Design review of the part built by this model. Coordinates are the model's own, in mm. A direction names the side the tool comes from. Give positions to 0.01 mm unless a question says otherwise; leave off trailing zeros. Order: outer loops, then holes, each group sorted by start corner. A loop starts at its lowest first (then second) coordinate and runs counter-clockwise, first axis right, second up. Notation, with made-up numbers: (42, -40) -> (50, -40) arc R17 ccw to (50, -33) -> close; hole circle Ø5 at (66.5, 56.5). An arc over 180 degrees is marked (long way). Return JSON: item names as keys, results as strings.
```python
from build123d import *

# Parameters (mm, degrees)
BOSS_EXTRUDE1_DEPTH = 176.53
BOSS_EXTRUDE2_DEPTH = 1.905


with BuildPart() as part:
    # Sketch2 → Boss-Extrude1 (new body)
    with BuildSketch(Plane.XY):
        with BuildLine():
            Line((-8.5725, 0), (8.5725, 0))
            ThreePointArc((8.5725, 0), (8.931710245, 0.148789755), (9.0805, 0.508))
            Line((9.0805, 0.508), (9.0805, 2.794))
            ThreePointArc((9.0805, 2.794), (8.931710245, 3.153210245), (8.5725, 3.302))
            Line((8.5725, 3.302), (5.9055, 3.302))
            Line((5.9055, 3.302), (5.9055, 2.5654))
            Line((5.9055, 2.5654), (7.8105, 2.5654))
            Line((7.8105, 2.5654), (7.8105, 1.2954))
            Line((7.8105, 1.2954), (-7.8105, 1.2954))
            Line((-7.8105, 1.2954), (-7.8105, 2.5654))
            Line((-7.8105, 2.5654), (-5.3975, 2.5654))
            Line((-5.3975, 2.5654), (-5.3975, 3.302))
            Line((-5.3975, 3.302), (-8.5725, 3.302))
            ThreePointArc((-8.5725, 3.302), (-8.931710245, 3.153210245), (-9.0805, 2.794))
            Line((-9.0805, 2.794), (-9.0805, 0.508))
            ThreePointArc((-9.0805, 0.508), (-8.931710245, 0.148789755), (-8.5725, 0))
        make_face()
    extrude(amount=-BOSS_EXTRUDE1_DEPTH)

    # Sketch3 → Boss-Extrude2 (add)
    with BuildSketch(Plane(origin=(0, 0, 0), x_dir=(1, 0, 0), z_dir=(0, 1, 0))):
        with BuildLine():
            Line((8.5725, 84.455), (8.5725, 92.075))
            ThreePointArc((8.5725, 92.075), (13.193617406, 88.265), (8.5725, 84.455))
        make_face()
    boss_extrude2 = extrude(amount=BOSS_EXTRUDE2_DEPTH)

    # Mirror1: Boss-Extrude2 across plane
    add(boss_extrude2.mirror(Plane(origin=(0, 0, 0), x_dir=(0, 0, 1), z_dir=(1, 0, 0))))


solid = part.part
```
Item 1: Machinability: for faces 1 (the face through (-7, 3.302, -87)), 2 (the face through (11, 1.905, -88)), 3 (the face through (-11, 1.905, -88)), which of the approach directions +Z, -Z, +X, -X, +Y, -Y give a long, thin tool a straight path to every point of the face, cutting with its end or side? Answer none if there is none.
Result set:
{"face 1": "+Z, -Z, +X, -X, +Y", "face 2": "+Z, -Z, +X, +Y", "face 3": "+Z, -Z, -X, +Y"}
Item 2: Add section A-A (z = -160). Give the boundary of the cut face in (x, y).
Result set:
{"outline": "(-9.08, 0.51) arc R0.51 ccw to (-8.57, 0) -> (8.57, 0) arc R0.51 ccw to (9.08, 0.51) -> (9.08, 2.79) arc R0.51 ccw to (8.57, 3.3) -> (5.91, 3.3) -> (5.91, 2.57) -> (7.81, 2.57) -> (7.81, 1.3) -> (-7.81, 1.3) -> (-7.81, 2.57) -> (-5.4, 2.57) -> (-5.4, 3.3) -> (-8.57, 3.3) arc R0.51 ccw to (-9.08, 2.79) -> close"}
Item 3: Add section C-C (x = -11.25). Give the boundary of the cut face in (y, z) (3 decimals).
Result set:
{"outline": "(0, -91.628) -> (1.905, -91.628) -> (1.905, -84.902) -> (0, -84.902) -> close"}
Item 4: For pin 1 (4.5 mm diameter, centred on x = 11.5, z = -90, fed in from +Y) (3 decimals); pin 2 (1.8 mm diameter, centred on y = 1.5, z = -119.5, fed in from -X); pin 3 (4.5 mm diameter, centred on x = 3.5, z = -117.5, fed in from +Y), all flat-tipped, find the tip position at first contact; note any pin that passes through.
Result set:
{"pin 1": "stops at y = 1.905", "pin 2": "stops at x = -9.08", "pin 3": "stops at y = 1.3"}
Item 5: Mouldability with a two-part tool opening along X and no side actions: class faces 4 (the face through (0, 0, -90)), 5 (the face through (0, 1.295, -87)) as released by +X, released by -X, zero draft, split by the parting line, or undercut.
Result set:
{"face 4": "zero draft", "face 5": "undercut"}
Item 6: Wall thickness on L1, parallel to X at y = 2.6, z = -88.5; L2, parallel to X at y = 2, z = -16; L3, parallel to Y at x = 7, z = -86: over which ranges is each line inside the solid? List them lowest first. Write a range as [from, to].
Result set:
{"L1": "x = [-9.08, -5.4], [5.91, 9.08]", "L2": "x = [-9.08, -7.81], [7.81, 9.08]", "L3": "y = [0, 1.3], [2.57, 3.3]"}
Item 7: Add section B-B (x = 3). Give the boundary of the cut face in (y, z).
Result set:
{"outline": "(0, -176.53) -> (1.3, -176.53) -> (1.3, 0) -> (0, 0) -> close"}
